Verification items for the finished model (mm, model axes). Face numbers are marked on the shaded views. A direction names the side the tool comes from. Give positions to 0.01 mm unless a question says otherwise; leave off trailing zeros. Write each loop counter-clockwise with the first axis right and the second up, starting at its lowest first coordinate (ties: lowest second). Pieces come first, ordered by that corner, then holes. Notation, with made-up numbers: (-20.75, 78.5) -> (5.25, 78.5) arc R22 ccw to (5.25, 101.5) -> close; hole circle Ø9 at (68, 54.25). An arc over 180 degrees is marked (long way). Write item = value, one per line.
from build123d import *

# Parameters (mm, degrees)
F0_W      = 77.7
F0_H      = 167.5
F1_DEPTH  = 33.34
F2_T      = -2
F3_R      = 10
F4_DEPTH  = 25
F5_W      = 77.7
F5_H      = 16
F6_DEPTH  = 3
F8_DEPTH  = 25
F9_W      = 77.7
F9_H      = 16
F10_DEPTH = 3
F12_DEPTH = 25
F13_W     = 14
F13_H     = 18
F14_DEPTH = 25


with BuildPart() as f1:
    # F0 (on Top) → F1 (new body)
    with BuildSketch(Plane.XY):
        Rectangle(F0_W, F0_H)
    extrude(amount=F1_DEPTH)

    # F2
    f2_openings = [f1.faces().sort_by_distance(p)[0] for p in [
        (0, 0, 0),
    ]]
    offset(amount=F2_T, openings=f2_openings)

    # F3 (on face) → F4 (cut)
    with BuildSketch(Plane(origin=(-38.85, 0, 0), x_dir=(0, -1, 0), z_dir=(-1, 0, 0))):
        with Locations((-19.975796, 16.67)):
            Circle(F3_R)
        with Locations((-48.75, 16.67)):
            Circle(F3_R)
    extrude(amount=-F4_DEPTH, mode=Mode.SUBTRACT)

    # F5 (on face) → F6 (join)
    with BuildSketch(Plane(origin=(0, 0, 0), x_dir=(1, 0, 0), z_dir=(0, 0, -1))):
        with Locations((0, 91.75)):
            Rectangle(F5_W, F5_H)
    extrude(amount=-F6_DEPTH)

    # F7 (on face) → F8 (cut)
    with BuildSketch(Plane.XY.offset(3)):
        with BuildLine():
            Line((-3.5, -87.75), (-3.5, -99.75))
            Line((-3.5, -99.75), (3.5, -99.75))
            Line((3.5, -99.75), (3.5, -87.75))
            ThreePointArc((3.5, -87.75), (2.62132, -85.62868), (0.5, -84.75))
            Line((0.5, -84.75), (-0.5, -84.75))
            ThreePointArc((-0.5, -84.75), (-2.62132, -85.62868), (-3.5, -87.75))
        make_face()
    extrude(amount=-F8_DEPTH, mode=Mode.SUBTRACT)

    # F9 (on face) → F10 (join)
    with BuildSketch(Plane(origin=(0, 0, 0), x_dir=(1, 0, 0), z_dir=(0, 0, -1))):
        with Locations((0, -91.75)):
            Rectangle(F9_W, F9_H)
    extrude(amount=-F10_DEPTH)

    # F11 (on face) → F12 (cut)
    with BuildSketch(Plane(origin=(0, 0, 0), x_dir=(1, 0, 0), z_dir=(0, 0, -1))):
        with BuildLine():
            Line((-3.5, -87.75), (-3.5, -99.75))
            Line((-3.5, -99.75), (3.5, -99.75))
            Line((3.5, -99.75), (3.5, -87.75))
            ThreePointArc((3.5, -87.75), (2.62132, -85.62868), (0.5, -84.75))
            Line((0.5, -84.75), (-0.5, -84.75))
            ThreePointArc((-0.5, -84.75), (-2.62132, -85.62868), (-3.5, -87.75))
        make_face()
    extrude(amount=-F12_DEPTH, mode=Mode.SUBTRACT)

    # F13 (on face) → F14 (cut)
    with BuildSketch(Plane(origin=(0, 99.75, 0), x_dir=(-1, 0, 0), z_dir=(0, 1, 0))):
        with Locations((18.85, 9)):
            Rectangle(F13_W, F13_H)
        with Locations((-18.85, 9)):
            Rectangle(F13_W, F13_H)
    extrude(amount=-F14_DEPTH, mode=Mode.SUBTRACT)


solid = f1.part
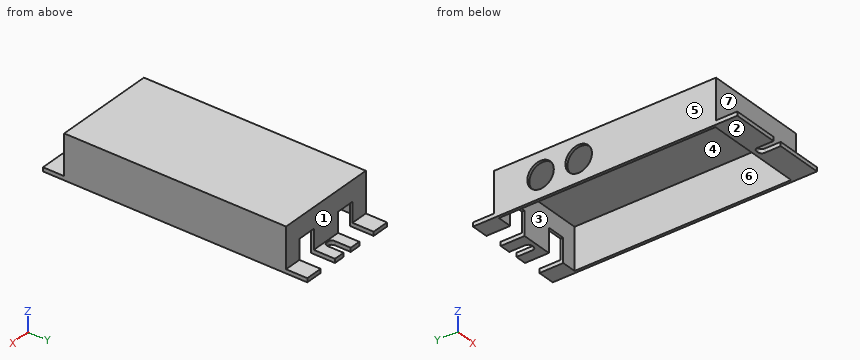
Item 1: Mould release check, pull along X, two halves, no side actions. Record for the marked faces 4, 5, 6 and 7: +X half, -X half, draft (parallel to the pull), parting line (faces both ways), or undercut.
Response values:
face_4 = undercut
face_5 = -X half
face_6 = undercut
face_7 = draft
Item 2: Go/stop test with flat-tipped pins: P1, Ø5.5, axis at y = 92.5, z = 6.5, coming from the -X side; P2, Ø15.5, axis at x = -9, z = 12, coming from the -Y side; P3, Ø10, axis at x = 13.5, y = -55, coming from the -Z side; P4, Ø1.1, axis at x = 0, z = 1.5, coming from the -Y side. Record where each tip stops, or that it passes through.
Response values:
P1 = through
P2 = -83.75
P3 = 31.34
P4 = -84.75
Item 3: Sectioned sample at A-A on y = 21. Record the cut outline in (x, z).
Response values:
outline = (-38.85, 0) -> (-36.85, 0) -> (-36.85, 6.72) -> (-38.85, 6.72) -> close; (-38.85, 26.62) -> (-36.85, 26.62) -> (-36.85, 31.34) -> (36.85, 31.34) -> (36.85, 0) -> (38.85, 0) -> (38.85, 33.34) -> (-38.85, 33.34) -> close
Item 4: Sectioned sample at B-B on z = 23. Record the cut outline in (x, y).
Response values:
outline = (-38.85, -83.75) -> (38.85, -83.75) -> (38.85, 83.75) -> (-38.85, 83.75) -> (-38.85, 56.49) -> (-36.85, 56.49) -> (-36.85, 81.75) -> (36.85, 81.75) -> (36.85, -81.75) -> (-36.85, -81.75) -> (-36.85, 12.23) -> (-38.85, 12.23) -> close; (-38.85, 27.72) -> (-36.85, 27.72) -> (-36.85, 41.01) -> (-38.85, 41.01) -> close
Item 5: Sectioned sample at D-D on y = 80. Record the cut outline in (x, z), then the cut area to 3 significant figures.
Response values:
outline = (-38.85, 0) -> (-36.85, 0) -> (-36.85, 31.34) -> (36.85, 31.34) -> (36.85, 0) -> (38.85, 0) -> (38.85, 33.34) -> (-38.85, 33.34) -> close
area = 281 mm^2
Item 6: Sectioned sample at C-C on x = 19. Record the cut outline in (y, z), then the cut area to 3 significant figures.
Response values:
outline = (-99.75, 0) -> (-81.75, 0) -> (-81.75, 31.34) -> (81.75, 31.34) -> (81.75, 18) -> (83.75, 18) -> (83.75, 33.34) -> (-83.75, 33.34) -> (-83.75, 3) -> (-99.75, 3) -> close
area = 472 mm^2
Item 7: Material ranges on line 1 (Y direction, x = 5.5, z = 13.5); line 2 (X direction, y = 77.5, z = 22); line 3 (Z direction, x = -37.5, y = 48.75), recorded low to high.
Response values:
line_1 = -83.75 to -81.75, 81.75 to 83.75
line_2 = -38.85 to -36.85, 36.85 to 38.85
line_3 = 0 to 6.67, 26.67 to 33.34
Item 8: Set-up check for the marked faces 1, 2 and 3: record each of +Z, -Z, +X, -X, +Y, -Y from which the full face is reachable in a straight line by a thin tool's end or side.
Response values:
face_1 = +Z, +X, -X, +Y
face_2 = -Z, +X, -X, +Y, -Y
face_3 = -Z
